The listing builds one solid part. Answer for the finished solid, in the listing's coordinates (mm). A direction names the side the tool comes from. Give positions to 0.01 mm unless a question says otherwise; leave off trailing zeros. Loops run counter-clockwise (first coordinate to the right, second up) from the corner with the lowest first, then second, coordinate; pieces in that order, holes last.
Item 1: Each of these flat-tipped pins is pushed along its axis until it touches: pin 1 Ø6 at (y, z) = (7, -18) entering from +X; pin 2 Ø1.5 at (x, y) = (20, 5) entering from +Z; pin 3 Ø3 at (y, z) = (10, -17.5) entering from +X. Where does it stop, or does it pass through?
Item 2: A tool of negligible diameter and unlimited length cuts with its end or side. For faces 5 (the face through (11, 9, 11)), 6 (the face through (-0.37, 5.42, -9.91)), from which of +Z, -Z, +X, -X, +Y, -Y can it reach the whole face along a straight path? Write none if from no direction.
Item 3: Section A-A, the plane z = 0 is taken. Give the vertices of the cut face in (x, y), and give its area (3 significant figures).
Item 4: Section D-D, the plane z = 8.25 is taken. Give the vertices of the cut face in (x, y).
Item 5: Section B-B, the plane y = 1.5 is taken. Give the number of separate pieces and of enclosed holes in the cut face, and give its area (3 significant figures).
Item 6: The mould has two halves that part along X. Classify faces 1 (the face through (31, 7.52, -9.76)), 2 (the face through (6.691, 10.014, 12.864)), 3 (the face through (-0.878, 5.423, -3.954)), 4 (the face through (-8, 0, -8)): pulls with the +X half, pulls with the -X half, needs draft (parallel to the pull), parting line crosses it, or undercut.
Item 7: Section C-C, the plane x = 8.25 is taken. Give the vertices of the cut face in (y, z), and give its area (3 significant figures).
Item 8: Consider line 1 along Z through (x, y) = (0, 6.7); line 2 along X through (y, z) = (4, -14); line 3 along Y through (x, z) = (-8, 21.5). Determine where each line is inside the solid, lowest interval first.
Autodesk Inventor part; units mm, degrees
ref_plane "YZ Plane" through (0, 0, 0) normal (1, 0, 0) x (0, 1, 0)
ref_plane "XZ Plane" through (0, 0, 0) normal (0, 1, 0) x (-1, 0, 0)
ref_plane "XY Plane" through (0, 0, 0) normal (0, 0, 1) x (1, 0, 0)
sketch "Boceto1" plane through (0, 0, 0) normal (0, 1, 0) x (-1, 0, 0)
  circle A0 centre (0, 0) radius 37
  dimension "d0" = 74
extrude "Extrusión1" add sketch "Boceto1" along normal blind 11
sketch "Boceto3" plane through (0, 0, 0) normal (0, -1, 0) x (1, 0, 0)
  circle A0 centre (0, 0) radius 8.25
  circle A1 centre (0, 8.25) radius 1.7
  circle A2 centre (8.25, 0) radius 1.7
  circle A3 centre (-8.25, 0) radius 1.7
  circle A4 centre (0, -8.25) radius 1.7
  dimension "d7" = 3.4
  dimension "d8" = 16.5
extrude "Extrusión3" cut sketch "Boceto3" against normal through all contours A0 A2 | A0 A2 | A1 A0 | A0 A1 | A4 A0 | A0 A4 | A3 A0 | A0 A3
sketch "Boceto5" plane through (0, 0, 0) normal (0, -1, 0) x (1, 0, 0)
  circle A0 centre (0, 0) radius 4.05
  dimension "d13" = 8.1
extrude "Extrusión5" cut sketch "Boceto5" against normal through all
sketch "Boceto8" plane through (0, 11, 0) normal (0, 1, 0) x (1, 0, 0)
  circle A0 centre (0, 0) radius 24.5
  circle A1 centre (0, 0) radius 37
  dimension "d25" = 49
  dimension "d26" = 74
extrude "Extrusión8" cut sketch "Boceto8" against normal blind 2
sketch "Boceto14" plane through (0, 9, 0) normal (0, 1, 0) x (1, 0, 0)
  circle A0 centre (0, 0) radius 28
  circle A1 centre (0, 28) radius 1.7
  circle A2 centre (-24.2487, 14) radius 1.7
  circle A3 centre (-24.2487, -14) radius 1.7
  circle A4 centre (0, -28) radius 1.7
  circle A5 centre (24.2487, -14) radius 1.7
  circle A6 centre (24.2487, 14) radius 1.7
  point P0 (-1.6992, -27.9484)
  point P1 (1.6992, -27.9484)
  dimension "d50" = 56
  dimension "d51" = 3.4
  dimension "d54" = 360
extrude "Extrusión12" cut sketch "Boceto14" against normal through all contours A6 A0 | A0 A6 | A5 A0 | A0 A5 | A1 A0 | A0 A1 | A4 A0 | A0 A4 | A2 A0 | A0 A2 | A3 A0 | A0 A3
sketch "Boceto15" plane through (0, 9, 0) normal (0, 1, 0) x (1, 0, 0)
  circle A0 centre (24.2487, 14) radius 1.7
  circle A1 centre (24.2487, 14) radius 3
  circle A2 centre (0, 28) radius 3
  circle A3 centre (-24.2487, 14) radius 3
  circle A4 centre (-24.2487, -14) radius 3
  circle A5 centre (0, -28) radius 3
  circle A6 centre (24.2487, -14) radius 3
  circle A7 centre (0, 0) radius 4.05
  circle A8 centre (0, 0) radius 32.5
  circle A9 centre (0, 0) radius 24.5
  dimension "d58" = 6
  dimension "d61" = 360
  dimension "d63" = 65
extrude "Extrusión13" cut sketch "Boceto15" against normal blind 3 contours A0 | A1 | A2 | A3 | A4 | A5 | A6 | A8
sketch "Boceto16" plane through (0, 11, 0) normal (0, 1, 0) x (1, 0, 0)
  circle A0 centre (0, 0) radius 14.5
  circle A1 centre (0, 0) radius 37
  dimension "d66" = 29
extrude "Extrusión14" cut sketch "Boceto16" against normal blind 2
equation "\"d1\" = Altura"
equation "\"Altura\" = 11"
properties part number "Joint - Primer segmento" material "Plastico PETG"
Worked answers:
1. pin 1: stops at x = 33.82
1. pin 2: stops at z = 31.6
1. pin 3: stops at x = 33.18
2. face 5: +Y
2. face 6: +Y, -Y
3. outline: (-37, 0) - (-9.95, 0) - (-9.95, 11) - (-14.5, 11) - (-14.5, 9) - (-24.5, 9) - (-24.5, 6) - (-32.5, 6) - (-32.5, 9) - (-37, 9) - close; (-6.55, 0) - (-4.05, 0) - (-4.05, 11) - (-6.55, 11) - close; (4.05, 0) - (6.55, 0) - (6.55, 11) - (4.05, 11) - close; (9.95, 0) - (37, 0) - (37, 9) - (32.5, 9) - (32.5, 6) - (24.5, 6) - (24.5, 9) - (14.5, 9) - (14.5, 11) - (9.95, 11) - close
3. area: 512 mm2
4. outline: (-36.07, 0) - (-1.7, 0) - (-1.7, 11) - (-11.92, 11) - (-11.92, 9) - (-23.07, 9) - (-23.07, 6) - (-31.44, 6) - (-31.44, 9) - (-36.07, 9) - close; (1.7, 0) - (36.07, 0) - (36.07, 9) - (31.44, 9) - (31.44, 6) - (23.07, 6) - (23.07, 9) - (11.92, 9) - (11.92, 11) - (1.7, 11) - close
5. separate pieces: 1
5. enclosed holes: 11
5. area: 4,160 mm2
6. face 1: undercut
6. face 2: parting line crosses it
6. face 3: undercut
6. face 4: needs draft
7. outline: (0, -36.07) - (9, -36.07) - (9, -31.44) - (6, -31.44) - (6, -23.07) - (9, -23.07) - (9, -11.92) - (11, -11.92) - (11, -1.7) - (0, -1.7) - close; (0, 1.7) - (11, 1.7) - (11, 11.92) - (9, 11.92) - (9, 23.07) - (6, 23.07) - (6, 31.44) - (9, 31.44) - (9, 36.07) - (0, 36.07) - close
7. area: 609 mm2
8. line 1: z = -37 to -32.5, -24.5 to -9.95, -6.55 to -4.05, 4.05 to 6.55, 9.95 to 24.5, 32.5 to 37
8. line 2: x = -34.25 to -25.95, -22.55 to 22.55, 25.95 to 34.25
8. line 3: y = 0 to 9
